from build123d import *

# Parameters (mm, degrees)
SKETCH1_W            = 43
SKETCH1_H            = 43
BOSS_EXTRUDE1_DEPTH  = 3
SKETCH2_R            = 3
SKETCH2_R_2          = 2
BOSS_EXTRUDE5_DEPTH  = 3
SKETCH2_9_R          = 3
SKETCH2_9_R_2        = 2
BOSS_EXTRUDE6_DEPTH  = 3
SKETCH2_10_R         = 3
SKETCH2_10_R_2       = 2
BOSS_EXTRUDE7_DEPTH  = 3
SKETCH2_11_R         = 3
SKETCH2_11_R_2       = 2
BOSS_EXTRUDE8_DEPTH  = 3
SKETCH3_W            = 4.5
SKETCH3_H            = 4
SKETCH3_R            = 1.5
BOSS_EXTRUDE9_DEPTH  = 2.5
FILLET2_R            = 2
SKETCH4_W            = 4.5
SKETCH4_H            = 4
SKETCH4_R            = 1.5
BOSS_EXTRUDE10_DEPTH = 2.5
FILLET3_R            = 2
SKETCH7_R            = 2
CUT_EXTRUDE1_DEPTH   = 65.142419661
SKETCH2_13_R         = 2
CUT_EXTRUDE2_DEPTH   = 65.142419661
SKETCH2_14_R         = 2
CUT_EXTRUDE3_DEPTH   = 65.142419661


with BuildPart() as part:
    # Sketch1 → Boss-Extrude1 (new body)
    with BuildSketch(Plane(origin=(0, 0, 0), x_dir=(1, 0, 0), z_dir=(0, 1, 0))):
        with Locations((21.5, 21.5)):
            Rectangle(SKETCH1_W, SKETCH1_H)
    extrude(amount=BOSS_EXTRUDE1_DEPTH)

    # Sketch2 → Boss-Extrude5 (add)
    with BuildSketch(Plane(origin=(0, 3, 0), x_dir=(1, 0, 0), z_dir=(0, 1, 0))):
        with Locations(Location((4, 39, 0), (0, 0, 90))):
            Circle(SKETCH2_R)
        with Locations(Location((4, 39, 0), (0, 0, 270))):
            Circle(SKETCH2_R_2, mode=Mode.SUBTRACT)
    extrude(amount=BOSS_EXTRUDE5_DEPTH)

    # Sketch2<9> → Boss-Extrude6 (add)
    with BuildSketch(Plane(origin=(0, 3, 0), x_dir=(1, 0, 0), z_dir=(0, 1, 0))):
        with Locations(Location((39, 39, 0), (0, 0, 90))):
            Circle(SKETCH2_9_R)
        with Locations(Location((39, 39, 0), (0, 0, 270))):
            Circle(SKETCH2_9_R_2, mode=Mode.SUBTRACT)
    extrude(amount=BOSS_EXTRUDE6_DEPTH)

    # Sketch2<10> → Boss-Extrude7 (add)
    with BuildSketch(Plane(origin=(0, 3, 0), x_dir=(1, 0, 0), z_dir=(0, 1, 0))):
        with Locations(Location((4, 4, 0), (0, 0, 90))):
            Circle(SKETCH2_10_R)
        with Locations(Location((4, 4, 0), (0, 0, 270))):
            Circle(SKETCH2_10_R_2, mode=Mode.SUBTRACT)
    extrude(amount=BOSS_EXTRUDE7_DEPTH)

    # Sketch2<11> → Boss-Extrude8 (add)
    with BuildSketch(Plane(origin=(0, 3, 0), x_dir=(1, 0, 0), z_dir=(0, 1, 0))):
        with Locations(Location((39, 4, 0), (0, 0, 90))):
            Circle(SKETCH2_11_R)
        with Locations(Location((39, 4, 0), (0, 0, 270))):
            Circle(SKETCH2_11_R_2, mode=Mode.SUBTRACT)
    extrude(amount=BOSS_EXTRUDE8_DEPTH)

    # Sketch3 → Boss-Extrude9 (add)
    with BuildSketch(Plane.XZ):
        with Locations((-2.25, -19.5)):
            Rectangle(SKETCH3_W, SKETCH3_H)
        with Locations(Location((-2.25, -19.5, 0), (0, 0, 270))):
            Circle(SKETCH3_R, mode=Mode.SUBTRACT)
    extrude(amount=-BOSS_EXTRUDE9_DEPTH)

    # Fillet2
    fillet2_edges = [part.edges().sort_by_distance(p)[0] for p in [
        (-4.5, 1.25, -21.5),
        (-4.5, 1.25, -17.5),
    ]]
    fillet(fillet2_edges, radius=FILLET2_R - 0.0001)  # a hair under: the kernel refuses the full size

    # Sketch4 → Boss-Extrude10 (add)
    with BuildSketch(Plane.XZ):
        with Locations((45.25, -19.5)):
            Rectangle(SKETCH4_W, SKETCH4_H)
        with Locations(Location((45.25, -19.5, 0), (0, 0, 270))):
            Circle(SKETCH4_R, mode=Mode.SUBTRACT)
    extrude(amount=-BOSS_EXTRUDE10_DEPTH)

    # Fillet3
    fillet3_edges = [part.edges().sort_by_distance(p)[0] for p in [
        (47.5, 1.25, -21.5),
        (47.5, 1.25, -17.5),
    ]]
    fillet(fillet3_edges, radius=FILLET3_R - 0.0001)  # a hair under: the kernel refuses the full size

    # Sketch7 → Cut-Extrude1 (cut, through all)
    with BuildSketch(Plane(origin=(0, 3, 0), x_dir=(1, 0, 0), z_dir=(0, 1, 0))):
        with Locations(Location((4, 39, 0), (0, 0, 270))):
            Circle(SKETCH7_R)
    extrude(amount=-CUT_EXTRUDE1_DEPTH, mode=Mode.SUBTRACT)

    # Sketch2<13> → Cut-Extrude2 (cut, through all)
    with BuildSketch(Plane(origin=(0, 3, 0), x_dir=(1, 0, 0), z_dir=(0, 1, 0))):
        with Locations(Location((39, 39, 0), (0, 0, 270))):
            Circle(SKETCH2_13_R)
    extrude(amount=-CUT_EXTRUDE2_DEPTH, mode=Mode.SUBTRACT)

    # Sketch2<14> → Cut-Extrude3 (cut, through all)
    with BuildSketch(Plane(origin=(0, 3, 0), x_dir=(1, 0, 0), z_dir=(0, 1, 0))):
        with Locations(Location((4, 4, 0), (0, 0, 270))):
            Circle(SKETCH2_14_R)
        with Locations(Location((39, 4, 0), (0, 0, 270))):
            Circle(SKETCH2_14_R)
    extrude(amount=-CUT_EXTRUDE3_DEPTH, mode=Mode.SUBTRACT)


solid = part.part
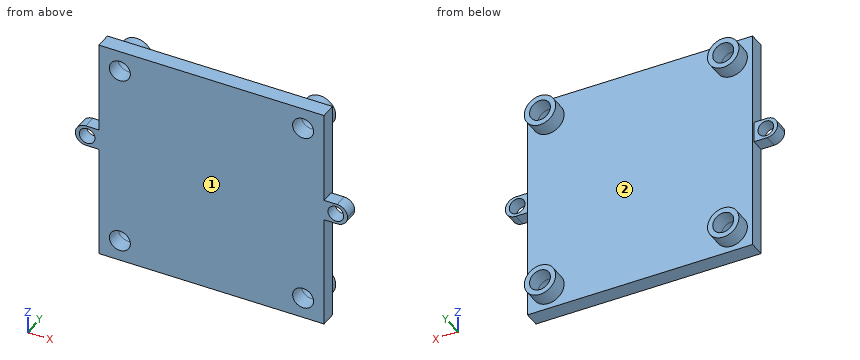
Work out the finished part from the listing and answer in its coordinate system (mm). Face numbers are marked on the shaded views. Coordinates: 2 decimals unless noted, no trailing zeros. Write each loop counter-clockwise with the first axis right and the second up, starting at its lowest first coordinate (ties: lowest second). Pieces come first, ordered by that corner, then holes. Notation, with made-up numbers: M 27.25,-22 L 61.25,-22 A23 ccw 61.25,2 Z; hole C 48.5,59.5 d3. An arc over 180 degrees is marked long. Write item = value, one per line.
1. The part is cut by section D-D (y = 1.5). State how many separate pieces and enclosed holes the cut face has, then the cut area to 3 significant figures.
Solution:
separate_pieces = 1
enclosed_holes = 6
area = 1,820 mm2
2. Flat-ended cylindrical pins translate along their axes: pin 1 (0.8 mm diameter, centred on x = 44, y = 1.5, fed in from +Z); pin 2 (3 mm diameter, centred on x = 4, z = -39, fed in from +Y) (1 decimal); pin 3 (4.5 mm diameter, centred on x = 45, z = -18.5, fed in from +Y); pin 4 (3 mm diameter, centred on x = 45, y = 1.5, fed in from -Z). Find the tip coordinate at first contact, or state that the pin passes through.
Solution:
pin_1 = -17.5
pin_2 = through
pin_3 = 3
pin_4 = -21.5
3. The part is cut by section A-A (y = 4.25). Determine the outline of the cut face in (x, z).
Solution:
outline = C 4,-39 d6; C 4,-4 d6; C 39,-39 d6; C 39,-4 d6; hole C 4,-39 d4; hole C 4,-4 d4; hole C 39,-39 d4; hole C 39,-4 d4
4. The part is cut by section C-C (x = 4). Determine the outline of the cut face in (y, z), then the cut area to 3 significant figures.
Solution:
outline = M 0,-43 L 3,-43 L 3,-42 L 6,-42 L 6,-41 L 0,-41 Z; M 0,-37 L 6,-37 L 6,-36 L 3,-36 L 3,-7 L 6,-7 L 6,-6 L 0,-6 Z; M 0,-2 L 6,-2 L 6,-1 L 3,-1 L 3,0 L 0,0 Z
area = 117 mm2
5. Determine the mould class of the marked faces 1 and 2 for opening direction Z: released by +Z, released by -Z, zero draft, split by the parting line, or undercut.
Solution:
face_1 = zero draft
face_2 = undercut
6. The part is cut by section B-B (z = -4). Determine the outline of the cut face in (x, y).
Solution:
outline = M 0,0 L 2,0 L 2,6 L 1,6 L 1,3 L 0,3 Z; M 6,0 L 37,0 L 37,6 L 36,6 L 36,3 L 7,3 L 7,6 L 6,6 Z; M 41,0 L 43,0 L 43,3 L 42,3 L 42,6 L 41,6 Z
7. Straight lines are drawn through the part: line 1 (X direction, y = 0.65, z = -4); line 2 (X direction, y = 4.65, z = -39); line 3 (Z direction, x = 40, y = 3.4). For each, find the intervals that lie inside material, in ascending order. Write a range as from..to.
Solution:
line_1 = 0..2, 6..37, 41..43
line_2 = 1..2, 6..7, 36..37, 41..42
line_3 = -41.83..-40.73, -37.27..-36.17, -6.83..-5.73, -2.27..-1.17
